```python
from build123d import *

# Parameters (mm, degrees)
SKETCH_1_W               = 82.4
SKETCH_1_H               = 6
EXTRUDE_1_DEPTH          = 2
SKETCH_2_W               = 2
SKETCH_2_H               = 6
EXTRUDE_2_DEPTH          = 10
CUT_EXTRUDE_1_REACH      = 85.485
SKETCH_3_R               = 1.25
CUT_EXTRUDE_2_DEPTH      = 84.221151158
CUT_EXTRUDE_2_DEPTH_BACK = 84.221151158
SKETCH_4_R               = 1.25
EXTRUDE_3_DEPTH          = 30
CUT_EXTRUDE_3_DEPTH      = 87.395370246
CUT_EXTRUDE_3_DEPTH_BACK = 87.395370246
SKETCH_9_R               = 1.25
SKETCH_10_R              = 1.25
CUT_EXTRUDE_4_DEPTH      = 89.25961704


with BuildPart() as part:
    # 草图1 → 凸台-拉伸1 (new body)
    with BuildSketch(Plane.XY):
        with Locations((41.2, 3)):
            Rectangle(SKETCH_1_W, SKETCH_1_H)
    extrude(amount=EXTRUDE_1_DEPTH)

    # 草图2 → 凸台-拉伸2 (add)
    with BuildSketch(Plane(origin=(0, 0, 0), x_dir=(-1, 0, 0), z_dir=(0, 0, -1))):
        with Locations((-1, 3)):
            Rectangle(SKETCH_2_W, SKETCH_2_H)
        with Locations((-81.4, 3)):
            Rectangle(SKETCH_2_W, SKETCH_2_H)
    extrude(amount=EXTRUDE_2_DEPTH)

    # 草图3 → 切除-拉伸1 (cut, up to next)
    with BuildSketch(Plane.XY.offset(2), mode=Mode.PRIVATE) as cut_extrude_1_sk1:
        with Locations((10, 3)):
            Circle(SKETCH_3_R)
    cut_extrude_1_tool1 = extrude(cut_extrude_1_sk1.sketch, amount=-CUT_EXTRUDE_1_REACH, mode=Mode.PRIVATE) & part.part
    # 草图3 → 切除-拉伸1 (cut, up to next)
    with BuildSketch(Plane.XY.offset(2), mode=Mode.PRIVATE) as cut_extrude_1_sk2:
        with Locations((72.4, 3)):
            Circle(SKETCH_3_R)
    cut_extrude_1_tool2 = extrude(cut_extrude_1_sk2.sketch, amount=-CUT_EXTRUDE_1_REACH, mode=Mode.PRIVATE) & part.part
    add(cut_extrude_1_tool1.solids().sort_by_distance((10, 3, 2))[0], mode=Mode.SUBTRACT)
    add(cut_extrude_1_tool2.solids().sort_by_distance((72.4, 3, 2))[0], mode=Mode.SUBTRACT)

    # 草图4 → 切除-拉伸2 (cut, two sides: drawn at the far end of the back side and taken through both)
    with BuildSketch(Plane(origin=(82.4, 0, 0), x_dir=(0, 0, -1), z_dir=(1, 0, 0)).offset(-CUT_EXTRUDE_2_DEPTH_BACK)):
        with Locations((5, 3)):
            Circle(SKETCH_4_R)
    extrude(amount=CUT_EXTRUDE_2_DEPTH + CUT_EXTRUDE_2_DEPTH_BACK, mode=Mode.SUBTRACT)

    # 草图5 → 凸台-拉伸3 (add)
    with BuildSketch(Plane.XZ):
        Polygon((0, 2), (0, -10), (2, -10), (2, 0), (80.4, 0), (80.4, -10), (82.4, -10), (82.4, 2), align=None)
    extrude(amount=EXTRUDE_3_DEPTH)

    # 草图9 → 切除-拉伸3 (cut, two sides: drawn at the far end of the back side and taken through both)
    with BuildSketch(Plane.ZY.offset(-80.4).offset(-CUT_EXTRUDE_3_DEPTH_BACK)):
        with Locations((-5, -21)):
            Circle(SKETCH_9_R)
    extrude(amount=CUT_EXTRUDE_3_DEPTH + CUT_EXTRUDE_3_DEPTH_BACK, mode=Mode.SUBTRACT)

    # 草图10 → 切除-拉伸4 (cut, through all)
    with BuildSketch(Plane(origin=(0, 0, 0), x_dir=(-1, 0, 0), z_dir=(0, 0, -1))):
        with Locations((-10, -21)):
            Circle(SKETCH_10_R)
        with Locations((-72, -21)):
            Circle(SKETCH_10_R)
    extrude(amount=-CUT_EXTRUDE_4_DEPTH, mode=Mode.SUBTRACT)


solid = part.part
```
Design review of the part built by this model. Coordinates are the model's own, in mm. A direction names the side the tool comes from. Coordinates: 2 decimals unless noted, no trailing zeros. Order: outer loops, then holes, each group sorted by start corner. A loop starts at its lowest first (then second) coordinate and runs counter-clockwise, first axis right, second up. Notation, with made-up numbers: M 72,-14.75 L 126,-14.75 A23 ccw 126,-5.75 Z; hole C 10,85.5 d9. An arc over 180 degrees is marked long. Answer as a JSON object with one key per item and string values. Group by question number.
1) Wall thickness on L1, parallel to Y at x = 81.5, z = -5; L2, parallel to X at y = -20.5, z = -1.5; L3, parallel to Z at x = 1.05, y = 3: over which ranges is each line inside the solid? List them lowest first.
2) Add section D-D, the plane y = -10. Write out the cut boundary in (x, z).
3) Tool access review of faces 1 (the flat face through (80.4, -12, -5)), 2 (the cylindrical face through (1.01, -22.22, -5.27)): name each direction out of +Z, -Z, +X, -X, +Y, -Y from which nothing blocks a thin tool from reaching the whole face with its end or side.
4) Add section C-C, the plane x = 10. Write out the cut boundary in (y, z).
5) Add section B-B, the plane y = -21. Write out the cut boundary in (x, z).
6) Mouldability with a two-part tool opening along Z and no side actions: class faces 3 (the flat face through (41, -12, 0)), 4 (the flat face through (2, -12, -5)), 5 (the cylindrical face through (0.99, 4.24, -4.84)) as pulls with the +Z half, pulls with the -Z half, needs draft (parallel to the pull), parting line crosses it, or undercut.
7) For pin 1 (2 mm diameter, centred on x = 8.5, y = 0, fed in from -Z); pin 2 (2 mm diameter, centred on x = 72, y = -21, fed in from +Z); pin 3 (3 mm diameter, centred on x = 10, y = -21, fed in from +Z), all flat-tipped, find the tip position at first contact; note any pin that passes through.
8) Add section A-A, the plane z = -8. Write out the cut boundary in (x, y).
Computed values:
{
 "1": {"L1": "y = -30 to -22.25, -19.75 to 1.75, 4.25 to 6", "L2": "x = 0 to 2, 80.4 to 82.4", "L3": "z = -10 to -6.25, -3.75 to 2"},
 "2": {"outline": "M 0,-10 L 2,-10 L 2,0 L 80.4,0 L 80.4,-10 L 82.4,-10 L 82.4,2 L 0,2 Z"},
 "3": {"face 1": "-Z, +Y, -Y", "face 2": "+X, -X"},
 "4": {"outline": "M -30,0 L -22.25,0 L -22.25,2 L -30,2 Z; M -19.75,0 L 1.75,0 L 1.75,2 L -19.75,2 Z; M 4.25,0 L 6,0 L 6,2 L 4.25,2 Z"},
 "5": {"outline": "M 0,-10 L 2,-10 L 2,-6.25 L 0,-6.25 Z; M 0,-3.75 L 2,-3.75 L 2,0 L 8.75,0 L 8.75,2 L 0,2 Z; M 11.25,0 L 70.75,0 L 70.75,2 L 11.25,2 Z; M 73.25,0 L 80.4,0 L 80.4,-3.75 L 82.4,-3.75 L 82.4,2 L 73.25,2 Z; M 80.4,-10 L 82.4,-10 L 82.4,-6.25 L 80.4,-6.25 Z"},
 "6": {"face 3": "pulls with the -Z half", "face 4": "needs draft", "face 5": "undercut"},
 "7": {"pin 1": "stops at z = 0", "pin 2": "passes through", "pin 3": "stops at z = 2"},
 "8": {"outline": "M 0,-30 L 2,-30 L 2,6 L 0,6 Z; M 80.4,-30 L 82.4,-30 L 82.4,6 L 80.4,6 Z"}
}
